```python
from build123d import *

# Parameters (mm, degrees)
PAD_DEPTH     = 51
THICKNESS_T   = -1
SKETCH001_W   = 2
SKETCH001_H   = 1
SKETCH001_W_2 = 1
SKETCH001_H_2 = 2
PAD001_DEPTH  = 50
FILLET_R      = 2
FILLET003_R   = 0.4


with BuildPart() as part:
    # Sketch → Pad (new body)
    with BuildSketch(Plane.XY):
        with BuildLine():
            Line((-33, 86.75), (33, 86.75))
            ThreePointArc((38, 81.75), (36.535534, 85.285534), (33, 86.75))
            Line((38, 81.75), (38, -81.75))
            ThreePointArc((33, -86.75), (36.535534, -85.285534), (38, -81.75))
            Line((33, -86.75), (-33, -86.75))
            ThreePointArc((-38, -81.75), (-36.535534, -85.285534), (-33, -86.75))
            Line((-38, -81.75), (-38, 81.75))
            ThreePointArc((-33, 86.75), (-36.535534, 85.285534), (-38, 81.75))
        make_face()
    extrude(amount=PAD_DEPTH)

    # Thickness
    thickness_openings = [part.faces().sort_by_distance(p)[0] for p in [
        (0, 0, 51),
    ]]
    offset(amount=THICKNESS_T, openings=thickness_openings)

    # Sketch001 (on Face19 of Thickness) → Pad001 (join)
    with BuildSketch(Plane.XY.offset(1)):
        with Locations((-36, 44.25)):
            Rectangle(SKETCH001_W, SKETCH001_H)
        with Locations((-36, 41.75)):
            Rectangle(SKETCH001_W, SKETCH001_H)
        with Locations((36, 44.25)):
            Rectangle(SKETCH001_W, SKETCH001_H)
        with Locations((36, 41.75)):
            Rectangle(SKETCH001_W, SKETCH001_H)
        with Locations((-36, -41.75)):
            Rectangle(SKETCH001_W, SKETCH001_H)
        with Locations((-36, -44.25)):
            Rectangle(SKETCH001_W, SKETCH001_H)
        with Locations((-36, 1.25)):
            Rectangle(SKETCH001_W, SKETCH001_H)
        with Locations((-36, -1.25)):
            Rectangle(SKETCH001_W, SKETCH001_H)
        with Locations((36, 1.25)):
            Rectangle(SKETCH001_W, SKETCH001_H)
        with Locations((36, -1.25)):
            Rectangle(SKETCH001_W, SKETCH001_H)
        with Locations((36, -41.75)):
            Rectangle(SKETCH001_W, SKETCH001_H)
        with Locations((36, -44.25)):
            Rectangle(SKETCH001_W, SKETCH001_H)
        with Locations((-1.25, -84.75)):
            Rectangle(SKETCH001_W_2, SKETCH001_H_2)
        with Locations((1.25, -84.75)):
            Rectangle(SKETCH001_W_2, SKETCH001_H_2)
        with Locations((-1.25, 84.75)):
            Rectangle(SKETCH001_W_2, SKETCH001_H_2)
        with Locations((1.25, 84.75)):
            Rectangle(SKETCH001_W_2, SKETCH001_H_2)
    extrude(amount=PAD001_DEPTH)

    # Fillet
    fillet_edges = [part.edges().sort_by_distance(p)[0] for p in [
        (0, 86.75, 0),
    ]]
    fillet(fillet_edges, radius=FILLET_R)

    # Fillet003
    fillet003_edges = [part.edges().sort_by_distance(p)[0] for p in [
        (1.75, -83.75, 26),
        (0.75, -83.75, 26),
        (-0.75, -83.75, 26),
        (-1.75, -83.75, 26),
        (35, 44.75, 26),
        (35, 43.75, 26),
        (35, 42.25, 26),
        (35, 41.25, 26),
        (35, 1.75, 26),
        (35, 0.75, 26),
        (35, -0.75, 26),
        (35, -1.75, 26),
        (35, -41.25, 26),
        (35, -42.25, 26),
        (35, -43.75, 26),
        (35, -44.75, 26),
        (-35, 44.75, 26),
        (-35, 43.75, 26),
        (-35, 42.25, 26),
        (-35, 41.25, 26),
        (-35, 1.75, 26),
        (-35, 0.75, 26),
        (-35, -0.75, 26),
        (-35, -1.75, 26),
        (-35, -41.25, 26),
        (-35, -42.25, 26),
        (-35, -43.75, 26),
        (-35, -44.75, 26),
        (1.75, 83.75, 26),
        (0.75, 83.75, 26),
        (-0.75, 83.75, 26),
        (-1.75, 83.75, 26),
    ]]
    fillet(fillet003_edges, radius=FILLET003_R)


with BuildPart() as part_1:
    # Body placement: moved
    add(part.part.moved(Location((0, 0, -295))))


solid = part_1.part
```
For this review, take the finished solid that the model builds, in its own axes (mm). A direction names the side the tool comes from. Coordinates: 2 decimals unless noted, no trailing zeros. Write each loop counter-clockwise with the first axis right and the second up, starting at its lowest first coordinate (ties: lowest second). Pieces come first, ordered by that corner, then holes. Notation, with made-up numbers: (70.25, -29.5) -> (109.25, -29.5) arc R27 ccw to (109.25, -5.5) -> close; hole circle Ø7 at (88.25, 28). An arc over 180 degrees is marked (long way). Put each result on its own line as item: value.
Q1. The part is to be moulded in two halves that separate along X. For faces 1 (the cylindrical face through (-35.859, -84.547, -269.35)), 2 (the flat face through (1, 1, -295)), 3 (the flat face through (38, 1, -269)), say which applies: +X half, -X half, draft (parallel to the pull), parting line (faces both ways), or undercut.
From the geometry:
face 1: undercut
face 2: draft
face 3: +X half
Q2. Take a section at B-B, the plane y = 49.5. State the section outline as (x, z) points, then the cut area to 3 significant figures.
From the geometry:
outline: (-38, -293) arc R2 ccw to (-36, -295) -> (36, -295) arc R2 ccw to (38, -293) -> (38, -244) -> (37, -244) -> (37, -294) -> (-37, -294) -> (-37, -244) -> (-38, -244) -> close
area: 174 mm2
Q3. Tool access review of faces 4 (the cylindrical face through (36.5, -85.32, -268.84)), 5 (the flat face through (18, -85.75, -269)): name each direction out of +Z, -Z, +X, -X, +Y, -Y from which nothing blocks a thin tool from reaching the whole face with its end or side.
From the geometry:
face 4: +Z, -Z, +X, -Y
face 5: +Z
Q4. Clearance check with flat-ended pins moving along their axes: pin 1 Ø1.3 at (y, z) = (84.5, -258) entering from +X; pin 2 Ø1.8 at (x, z) = (36.5, -277) entering from +Y; pin 3 Ø0.5 at (x, z) = (36.5, -271) entering from -Y. State where each tip first meets the part, or that it passes through.
From the geometry:
pin 1: stops at x = 37.54
pin 2: stops at y = 86.02
pin 3: stops at y = -85.55
Q5. Take a section at A-A, the plane x = 29.5. State the section outline as (y, z) points.
From the geometry:
outline: (-86.75, -293) arc R2 ccw to (-84.75, -295) -> (84.75, -295) arc R2 ccw to (86.75, -293) -> (86.75, -244) -> (85.75, -244) -> (85.75, -294) -> (-85.75, -294) -> (-85.75, -244) -> (-86.75, -244) -> close
Q6. Wall thickness on L1, parallel to X at y = 48, z = -252; L2, parallel to Y at x = 27, z = -291.5; L3, parallel to Z at x = -25.5, y = 50: over which ranges is each line inside the solid? List them lowest first.
From the geometry:
L1: x = -38 to -37, 37 to 38
L2: y = -86.75 to -85.75, 85.75 to 86.75
L3: z = -295 to -294
